Could you check a few things on this model? Use its own coordinates, in mm. A direction names the side the tool comes from. Coordinates: 2 decimals unless noted, no trailing zeros. Loops run counter-clockwise (first coordinate to the right, second up) from the corner with the lowest first, then second, coordinate; pieces in that order, holes last. Notation, with made-up numbers: (-35, 67) - (7, 67) arc R19 ccw to (7, 96) - close; hole circle Ø5 at (-40, 66.25). An arc over 180 degrees is marked (long way). One line per question, with ' | ' between items. Start each with the question number.
1. I want a section at A-A, the plane x = 0. Write out the boundary of the cut face in (y, z).
2. I'm going to push flat-ended pins straight in: P1, Ø6.5, axis at y = 0, z = -19.05, coming from the +X side; P2, Ø3.5, axis at y = 0, z = -19.05, coming from the +X side. Where does each tip first touch, or does it pass through?
3. Please list where these lines run through material, in increasing order: L1, parallel to Z at x = 0, y = 0; L2, parallel to Z at x = -18, y = 0; L3, parallel to Y at x = -15, z = 19. Write a range as [from, to].
4. Which directions (+Z, -Z, +X, -X, +Y, -Y) give clear straight access to the entire face, cutting with the end or side of a thin tool? Please do faces 5 (the cylindrical face through (18.688, -0.089, -17.033)), 6 (the cylindrical face through (-4.395, 0.086, -68.775)), 7 (the cylindrical face through (-18.688, -0.607, 17.124)).
5. We'd pull the mould along Y, two halves only. Please class faces 1 (the cylindrical face through (-1.25, -0.09, 21.37)), 2 (the conical face through (-10.78, -0.11, -19.38)), 3 (the flat face through (0, -6.16, -1)), 4 (the conical face through (10.78, -0.11, -19.38)): pulls with the +Y half, pulls with the -Y half, needs draft (parallel to the pull), parting line crosses it, or undercut.
6. I want a section at B-B, the plane y = -4.25. Count the separate pieces of the cut face and the enclosed holes in it, then the cut area to 3 significant figures.
from build123d import *

# Parameters (mm, degrees)
SKETCH1_W                       = 50.8
SKETCH1_H                       = 152.4
EXTRUDE1_DEPTH                  = 6.1595
CUT_EXTRUDE1_REACH              = 14.319
SKETCH2_R                       = 9.525
F_1_2_20_TAPPED_HOLE1_D         = 11.50874
F_1_2_20_TAPPED_HOLE1_DEPTH     = 12.319
F_10_32_TAPPED_HOLE1_AT_2_COUNT = 2
F_10_32_TAPPED_HOLE1_AT_2_PITCH = 38.1


with BuildPart() as part:
    # Sketch1 → Extrude1 (new body, symmetric)
    with BuildSketch(Plane(origin=(0, 0, 0), x_dir=(1, 0, 0), z_dir=(0, 1, 0))):
        Rectangle(SKETCH1_W, SKETCH1_H)
    extrude(amount=EXTRUDE1_DEPTH, both=True)

    # Sketch2 → Cut-Extrude1 (cut, up to next)
    with BuildSketch(Plane(origin=(0, 6.1595, 0), x_dir=(-1, 0, 0), z_dir=(0, 1, 0)), mode=Mode.PRIVATE) as cut_extrude1_sk1:
        with Locations((0, -60.325)):
            Circle(SKETCH2_R)
    cut_extrude1_tool1 = extrude(cut_extrude1_sk1.sketch, amount=-CUT_EXTRUDE1_REACH, mode=Mode.PRIVATE) & part.part
    add(cut_extrude1_tool1.solids().sort_by_distance((0, 6.1595, -60.325))[0], mode=Mode.SUBTRACT)
    # Sketch2 → Cut-Extrude1 (cut, up to next)
    with BuildSketch(Plane(origin=(0, 6.1595, 0), x_dir=(-1, 0, 0), z_dir=(0, 1, 0)), mode=Mode.PRIVATE) as cut_extrude1_sk2:
        with Locations((0, 60.325)):
            Circle(SKETCH2_R)
    cut_extrude1_tool2 = extrude(cut_extrude1_sk2.sketch, amount=-CUT_EXTRUDE1_REACH, mode=Mode.PRIVATE) & part.part
    add(cut_extrude1_tool2.solids().sort_by_distance((0, 6.1595, 60.325))[0], mode=Mode.SUBTRACT)

    # 1/2-20 Tapped Hole1
    with Locations(Plane(origin=(0, 6.1595, 0), x_dir=(-1, 0, 0), z_dir=(0, 1, 0))):
        with Locations((0, -26.9875), (0, 26.9875)):
            Hole(F_1_2_20_TAPPED_HOLE1_D / 2, depth=F_1_2_20_TAPPED_HOLE1_DEPTH)

    # Sketch10 → #10-32 Tapped Hole1 (revolve, cut)
    with BuildSketch(Plane(origin=(25.4, 0, 19.05), x_dir=(0, 0, -1), z_dir=(0, 1, 0))):
        Polygon((0, 0), (0, 14.827717848), (2.0193, 13.6144), (2.0193, 0), align=None)
    f_10_32_tapped_hole1 = revolve(axis=Axis((31.75, 0, 19.05), (-1, 0, 0)), mode=Mode.SUBTRACT)

    # #10-32 Tapped Hole1 at 2: #10-32 Tapped Hole1 ×2
    with Locations(*[(0, 0, -i * F_10_32_TAPPED_HOLE1_AT_2_PITCH) for i in range(1, F_10_32_TAPPED_HOLE1_AT_2_COUNT)]):
        add(f_10_32_tapped_hole1, mode=Mode.SUBTRACT)

    # Mirror1: #10-32 Tapped Hole1 across plane
    add(f_10_32_tapped_hole1.mirror(Plane(origin=(0, 0, 0), x_dir=(0, 0, 1), z_dir=(1, 0, 0))), mode=Mode.SUBTRACT)

    # Mirror1 copy 1 sketch → Mirror1 copy 1 (revolve, cut)
    with BuildSketch(Plane(origin=(-25.4, 0, -19.05), x_dir=(0, 0, -1), z_dir=(0, 1, 0))):
        Polygon((0, 0), (0, -14.827717848), (2.0193, -13.6144), (2.0193, 0), align=None)
    revolve(axis=Axis((-31.75, 0, -19.05), (-1, 0, 0)), mode=Mode.SUBTRACT)


solid = part.part
Results are:
1) outline: (-6.16, -76.2) - (6.16, -76.2) - (6.16, -69.85) - (-6.16, -69.85) - close; (-6.16, -50.8) - (6.16, -50.8) - (6.16, -32.74) - (-6.16, -32.74) - close; (-6.16, -21.23) - (6.16, -21.23) - (6.16, 21.23) - (-6.16, 21.23) - close; (-6.16, 32.74) - (6.16, 32.74) - (6.16, 50.8) - (-6.16, 50.8) - close; (-6.16, 69.85) - (6.16, 69.85) - (6.16, 76.2) - (-6.16, 76.2) - close
2) P1: stops at x = 25.4 | P2: stops at x = 11.62
3) L1: z = [-76.2, -69.85], [-50.8, -32.74], [-21.23, 21.23], [32.74, 50.8], [69.85, 76.2] | L2: z = [-76.2, -21.07], [-17.03, 17.03], [21.07, 76.2] | L3: y = [-6.16, -2.02], [2.02, 6.16]
4) face 5: +X | face 6: +Y, -Y | face 7: -X
5) face 1: needs draft | face 2: undercut | face 3: pulls with the -Y half | face 4: undercut
6) separate pieces: 1 | enclosed holes: 4 | area: 6,960 mm2
